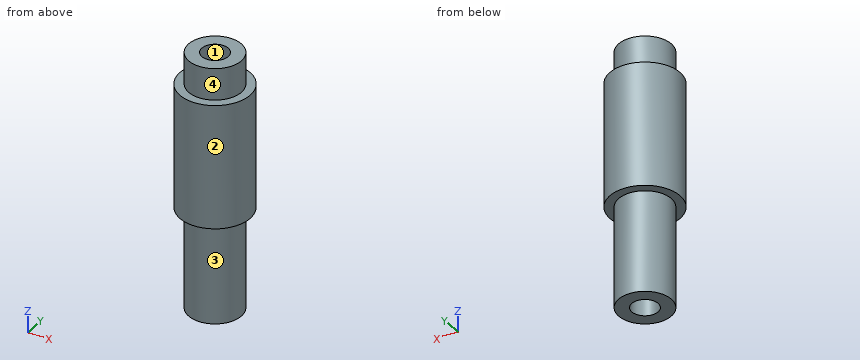
```python
from build123d import *

# Parameters (mm, degrees)
SKETCH_1_R          = 4
SKETCH_1_R_2        = 1.5
EXTRUDE_3_DEPTH     = 29.2
SKETCH_3_R          = 4
SKETCH_3_R_2        = 3
CUT_EXTRUDE_1_DEPTH = 11.5
CUT_EXTRUDE_START   = -3.6
SKETCH_4_R          = 4
SKETCH_4_R_2        = 3
CUT_EXTRUDE_2_DEPTH = 3.6


with BuildPart() as part:
    # ｽｹｯﾁ1 → ﾎﾞｽ - 押し出し3 (new body)
    with BuildSketch(Plane.XY):
        with Locations(Location((0, 0, 0), (0, 0, 180))):
            Circle(SKETCH_1_R)
        with Locations(Location((0, 0, 0), (0, 0, 180))):
            Circle(SKETCH_1_R_2, mode=Mode.SUBTRACT)
    extrude(amount=EXTRUDE_3_DEPTH)

    # ｽｹｯﾁ3 → ｶｯﾄ - 押し出し1 (cut)
    with BuildSketch(Plane(origin=(0, 0, 0), x_dir=(-1, 0, 0), z_dir=(0, 0, -1))):
        Circle(SKETCH_3_R)
        Circle(SKETCH_3_R_2, mode=Mode.SUBTRACT)
    extrude(amount=-CUT_EXTRUDE_1_DEPTH, mode=Mode.SUBTRACT)

    # ｽｹｯﾁ4 → ｶｯﾄ - 押し出し2 (cut)
    with BuildSketch(Plane.XY.offset(29.2).offset(CUT_EXTRUDE_START)):
        with Locations(Location((0, 0, 0), (0, 0, 180))):
            Circle(SKETCH_4_R)
        with Locations(Location((0, 0, 0), (0, 0, 180))):
            Circle(SKETCH_4_R_2, mode=Mode.SUBTRACT)
    extrude(amount=CUT_EXTRUDE_2_DEPTH, mode=Mode.SUBTRACT)


solid = part.part
```
The listing builds one solid part. Answer for the finished solid, in the listing's coordinates (mm). Face numbers are marked on the shaded views. A direction names the side the tool comes from. Round coordinates to 2 decimals unless told otherwise and drop trailing zeros. Write each loop counter-clockwise with the first axis right and the second up, starting at its lowest first coordinate (ties: lowest second). Pieces come first, ordered by that corner, then holes. Notation, with made-up numbers: (32, -38) -> (48, -38) arc R34 cw to (48, -8) -> close; hole circle Ø3 at (-35, 88). An arc over 180 degrees is marked (long way). Use CSV: the item, a comma, the result in double quotes. Start each with the question number.
(1) The mould has two halves that part along X. Classify the marked faces 1 and 2: released by +X, released by -X, zero draft, split by the parting line, or undercut.
(2) Each of these flat-tipped pins is pushed along its axis until it touches: pin 1 (1.5 mm diameter, centred on y = -1.5, z = 4.5, fed in from +X); pin 2 (2.5 mm diameter, centred on x = 0, y = 0, fed in from +Z) (3 decimals); pin 3 (3 mm diameter, centred on y = -2.5, z = 25.5, fed in from -X); pin 4 (2 mm diameter, centred on y = -2, z = 24.5, fed in from +X). Where does it stop, or does it pass through?
(3) Section D-D on y = 2.5 is taken. Give the vertices of the cut face in (x, z).
(4) Which of the six approach directions +Z, -Z, +X, -X, +Y, -Y give full straight-line access (tool end or side, diameter ignored) to the marked faces 3 and 4?
(5) Consider L1, parallel to Y at x = 0, z = 21.25; L2, parallel to Y at x = 0, z = 10.75; L3, parallel to Z at x = 3, y = 2.5. Determine where each line is inside the solid, lowest interval first. Write a range as from..to.
(6) Section C-C on z = 3.75 is taken. Give the vertices of the cut face in (x, y), then the cut area to 3 significant figures.
(7) Section A-A on y = 0 is taken. Give the vertices of the cut face in (x, z), then the cut area to 3 significant figures.
A:
1,face 1,"undercut"
1,face 2,"split by the parting line"
2,pin 1,"stops at x = 2.9"
2,pin 2,"passes through"
2,pin 3,"stops at x = -3.87"
2,pin 4,"stops at x = 3.87"
3,outline,"(-3.12, 11.5) -> (-1.66, 11.5) -> (-1.66, 0) -> (1.66, 0) -> (1.66, 11.5) -> (3.12, 11.5) -> (3.12, 25.6) -> (1.66, 25.6) -> (1.66, 29.2) -> (-1.66, 29.2) -> (-1.66, 25.6) -> (-3.12, 25.6) -> close"
4,face 3,"-Z"
4,face 4,"+Z"
5,L1,"y = -4..-1.5, 1.5..4"
5,L2,"y = -3..-1.5, 1.5..3"
5,L3,"z = 11.5..25.6"
6,outline,"circle Ø6 at (0, 0); hole circle Ø3 at (0, 0)"
6,area,"21.2 mm²"
7,outline,"(-4, 11.5) -> (-3, 11.5) -> (-3, 0) -> (-1.5, 0) -> (-1.5, 29.2) -> (-3, 29.2) -> (-3, 25.6) -> (-4, 25.6) -> close; (1.5, 0) -> (3, 0) -> (3, 11.5) -> (4, 11.5) -> (4, 25.6) -> (3, 25.6) -> (3, 29.2) -> (1.5, 29.2) -> close"
7,area,"116 mm²"
